from build123d import *

# Parameters (mm, degrees)
SKETCH1_R                = 13.85
BOSS_EXTRUDE1_DEPTH      = 26
CHAMFER1_SIZE            = 1.5
CHAMFER2_SIZE            = 3
SKETCH2_R                = 4.5
BOSS_EXTRUDE2_DEPTH      = 4
SKETCH3_R                = 1.585
BOSS_EXTRUDE3_DEPTH      = 10
M3_CLEARANCE_HOLE1_D     = 3.4
M3_CLEARANCE_HOLE1_DEPTH = 10
M3_CLEARANCE_HOLE1_TIP   = 1.021463052
M2_CLEARANCE_HOLE1_D     = 2.4
M2_CLEARANCE_HOLE1_DEPTH = 10
M2_CLEARANCE_HOLE1_TIP   = 0.721032743


with BuildPart() as part:
    # Sketch1 → Boss-Extrude1 (new body)
    with BuildSketch(Plane.XY):
        with Locations(Location((0, 0, 0), (0, 0, 180))):
            Circle(SKETCH1_R)
    extrude(amount=BOSS_EXTRUDE1_DEPTH)

    # Chamfer1
    chamfer1_edges = [part.edges().sort_by_distance(p)[0] for p in [
        (13.85, 0, 26),
    ]]
    chamfer(chamfer1_edges, length=CHAMFER1_SIZE)

    # Chamfer2
    chamfer2_edges = [part.edges().sort_by_distance(p)[0] for p in [
        (13.85, 0, 0),
    ]]
    chamfer(chamfer2_edges, length=CHAMFER2_SIZE)

    # Sketch2 → Boss-Extrude2 (add)
    with BuildSketch(Plane(origin=(0, 0, 0), x_dir=(-1, 0, 0), z_dir=(0, 0, -1))):
        Circle(SKETCH2_R)
    extrude(amount=BOSS_EXTRUDE2_DEPTH)

    # Sketch3 → Boss-Extrude3 (add)
    with BuildSketch(Plane.XY.offset(26)):
        Circle(SKETCH3_R)
    extrude(amount=BOSS_EXTRUDE3_DEPTH)

    # M3 Clearance Hole1
    with Locations(Plane.XY.offset(26)):
        with Locations((-5.656854249, 5.656854249), (6.717514421, 6.717514421), (5.656854249, -5.656854249), (-6.717514421, -6.717514421)):
            Hole(M3_CLEARANCE_HOLE1_D / 2, depth=M3_CLEARANCE_HOLE1_DEPTH)
            with Locations((0, 0, -(M3_CLEARANCE_HOLE1_DEPTH + M3_CLEARANCE_HOLE1_TIP / 2))):  # 118° drill point
                Cone(0, M3_CLEARANCE_HOLE1_D / 2, M3_CLEARANCE_HOLE1_TIP, mode=Mode.SUBTRACT)

    # M2 Clearance Hole1
    with Locations(Plane(origin=(0, 0, 0), x_dir=(-1, 0, 0), z_dir=(0, 0, -1))):
        with Locations((0, 6), (5.196152423, -3), (-5.196152423, -3)):
            Hole(M2_CLEARANCE_HOLE1_D / 2, depth=M2_CLEARANCE_HOLE1_DEPTH)
            with Locations((0, 0, -(M2_CLEARANCE_HOLE1_DEPTH + M2_CLEARANCE_HOLE1_TIP / 2))):  # 118° drill point
                Cone(0, M2_CLEARANCE_HOLE1_D / 2, M2_CLEARANCE_HOLE1_TIP, mode=Mode.SUBTRACT)


solid = part.part
CAD build for the part. Positions are in the model's coordinates, mm. A direction names the side the tool comes from. Coordinates: 2 decimals unless noted, no trailing zeros. Order: outer loops, then holes, each group sorted by start corner. A loop starts at its lowest first (then second) coordinate and runs counter-clockwise, first axis right, second up. Notation, with made-up numbers: (83.5, 44.25) -> (118.5, 44.25) arc R23 cw to (118.5, 65.25) -> close; hole circle Ø9 at (-6, 29.25). An arc over 180 degrees is marked (long way). Answer in a Markdown table with one row per item.
1) Band-saw the part on D-D (z = 26.5). List the corners of the cut face in (x, y) (3 decimals).
Check values:
| item | result |
|---|---|
| outline | circle Ø3.17 at (0, 0) |
2) Mould opens along Y. For faces 1 (the face through (4.086, -6.308, 20.93)), 2 (the face through (0, 0, 36)), 3 (the face through (-6.952, -6.897, 15.156)), 4 (the face through (-5.07, 9.76, 0.15)) say: pulls with the +Y half, pulls with the -Y half, needs draft (parallel to the pull), parting line crosses it, or undercut.
Check values:
| item | result |
|---|---|
| face 1 | undercut |
| face 2 | needs draft |
| face 3 | undercut |
| face 4 | parting line crosses it |
3) Band-saw the part on C-C (z = 6.5). List the corners of the cut face in (x, y), and give its area (3 significant figures).
Check values:
| item | result |
|---|---|
| outline | circle Ø27.7 at (0, 0); hole circle Ø2.4 at (-5.2, -3); hole circle Ø2.4 at (0, 6); hole circle Ø2.4 at (5.2, -3) |
| area | 589 mm2 |
4) Which spindle directions (+Z, -Z, +X, -X, +Y, -Y) get a long thin tool onto all of the face, cutting with end or side? Do faces 5 (the face through (0.59, 4.46, -1.97)), 6 (the face through (-7.631, -5.284, 20.93)), 7 (the face through (0, 0, -4)). Say none if no direction does.
Check values:
| item | result |
|---|---|
| face 5 | -Z |
| face 6 | +Z |
| face 7 | -Z, +X, -X, +Y, -Y |
5) Flat gauge pins, fed straight in: P1, Ø2, axis at x = 5.2, y = -3, coming from the -Z side; P2, Ø3, axis at x = -6.72, y = -6.72, coming from the +Z side; P3, Ø8, axis at x = -0.5, y = -8, coming from the +Z side. Where does each tip first touch, or does it go through?
Check values:
| item | result |
|---|---|
| P1 | z = 10.12 |
| P2 | z = 15.88 |
| P3 | z = 26 |
6) Drill centre lines: line 1 (X direction, y = -3, z = 5); line 2 (X direction, y = -3, z = 2); line 3 (Z direction, x = -1.25, y = -5). Where is each one in solid material? Low to high.
Check values:
| item | result |
|---|---|
| line 1 | -13.52 to -6.4, -4 to 4, 6.4 to 13.52 |
| line 2 | -12.49 to -6.4, -4 to 4, 6.4 to 12.49 |
| line 3 | 0 to 26 |
7) Band-saw the part on A-A (y = 0). List the corners of the cut face in (x, z) (3 decimals), and give its area (3 significant figures).
Check values:
| item | result |
|---|---|
| outline | (-13.85, 3) -> (-10.85, 0) -> (-4.5, 0) -> (-4.5, -4) -> (4.5, -4) -> (4.5, 0) -> (10.85, 0) -> (13.85, 3) -> (13.85, 24.5) -> (12.35, 26) -> (1.585, 26) -> (1.585, 36) -> (-1.585, 36) -> (-1.585, 26) -> (-12.35, 26) -> (-13.85, 24.5) -> close |
| area | 777 mm2 |
8) Band-saw the part on B-B (z = 22). List the corners of the cut face in (x, y).
Check values:
| item | result |
|---|---|
| outline | circle Ø27.7 at (0, 0); hole circle Ø3.4 at (-6.72, -6.72); hole circle Ø3.4 at (-5.66, 5.66); hole circle Ø3.4 at (5.66, -5.66); hole circle Ø3.4 at (6.72, 6.72) |
